Autodesk Inventor part; units mm, degrees
ref_plane "YZ Plane" through (0, 0, 0) normal (1, 0, 0) x (0, 1, 0)
ref_plane "XZ Plane" through (0, 0, 0) normal (0, 1, 0) x (-1, 0, 0)
ref_plane "XY Plane" through (0, 0, 0) normal (0, 0, 1) x (1, 0, 0)
sketch "Sketch1" plane through (0, 0, 0) normal (0, 0, 1) x (1, 0, 0)
  circle A0 centre (0, 0) radius 51.6188
  dimension "d0" = 103.2376
extrude "Extrusion1" add sketch "Sketch1" along normal mid plane 10
sketch "Sketch2" plane through (0, 0, 5) normal (0, 0, 1) x (1, 0, 0)
  circle A0 centre (0, 0) radius 51.6188
  arc A1 (-32.3092, 40.2568) -> (32.3092, 40.2568) centre (0, 73) ccw
  line L0 (0, 0) -> (36.5, 36.5) construction
  line L1 (0, -76.5426) -> (0, 97.9238) construction
  arc A2 (11.5258, 16.7584) -> (16.7584, 11.5258) centre (14.1421, 14.1421) ccw
  line L2 (11.5258, 16.7584) -> (33.7898, 39.0224)
  line L3 (16.7584, 11.5258) -> (39.0224, 33.7898)
  dimension "d3" = 46
  dimension "d4" = 73
  dimension "d5" = 20
  dimension "d6" = 45
  dimension "d7" = 3.7
extrude "Extrusion2" cut sketch "Sketch2" against normal through all contours L3 A2 L2 A0 | A0 A1
pattern_circular "Circular Pattern1" count 4 over 360 about axis through (0, 0, 0) along (0, 0, 1) of "Extrusion2"
chamfer "Chamfer1" distance 0.5 angle 45 8 edges at (0, 27, -5) (0, 27, 5) (27, 0, 5) (27, 0, -5) (-27, 0, 5) (0, -27, 5) (-27, 0, -5) (0, -27, -5)
sketch "Sketch3" plane through (0, 0, 5) normal (0, 0, 1) x (1, 0, 0)
  arc A0 (32.7, -39.9401) -> (-32.7, -39.9401) centre (0, -73) ccw
  line L0 (33.7898, -39.0224) -> (11.5258, -16.7584)
  arc A1 (16.7584, -11.5258) -> (11.5258, -16.7584) centre (14.1421, -14.1421) ccw
  line L1 (16.7584, -11.5258) -> (39.0224, -33.7898)
  arc A2 (39.9401, 32.7) -> (39.9401, -32.7) centre (73, 0) ccw
  line L2 (39.0224, 33.7898) -> (16.7584, 11.5258)
  arc A3 (11.5258, 16.7584) -> (16.7584, 11.5258) centre (14.1421, 14.1421) ccw
  line L3 (11.5258, 16.7584) -> (33.7898, 39.0224)
  arc A4 (-32.7, 39.9401) -> (32.7, 39.9401) centre (0, 73) ccw
  line L4 (-33.7898, 39.0224) -> (-11.5258, 16.7584)
  arc A5 (-16.7584, 11.5258) -> (-11.5258, 16.7584) centre (-14.1421, 14.1421) ccw
  line L5 (-16.7584, 11.5258) -> (-39.0224, 33.7898)
  arc A6 (-39.9401, -32.7) -> (-39.9401, 32.7) centre (-73, 0) ccw
  line L6 (-39.0224, -33.7898) -> (-16.7584, -11.5258)
  arc A7 (-11.5258, -16.7584) -> (-16.7584, -11.5258) centre (-14.1421, -14.1421) ccw
  line L7 (-11.5258, -16.7584) -> (-33.7898, -39.0224)
  line L8 (14.843, 22.904) -> (10.1116, 18.1726)
  arc A8 (10.1116, 18.1726) -> (18.1726, 10.1116) centre (14.1421, 14.1421) ccw
  line L9 (18.1726, 10.1116) -> (22.904, 14.843)
  arc A9 (26.2462, 12.8969) -> (26.2462, -12.8969) centre (73, 0) ccw
  line L10 (22.904, -14.843) -> (18.1726, -10.1116)
  arc A10 (18.1726, -10.1116) -> (10.1116, -18.1726) centre (14.1421, -14.1421) ccw
  line L11 (10.1116, -18.1726) -> (14.843, -22.904)
  arc A11 (12.8969, -26.2462) -> (-12.8969, -26.2462) centre (0, -73) ccw
  line L12 (-14.843, -22.904) -> (-10.1116, -18.1726)
  arc A12 (-10.1116, -18.1726) -> (-18.1726, -10.1116) centre (-14.1421, -14.1421) ccw
  line L13 (-18.1726, -10.1116) -> (-22.904, -14.843)
  arc A13 (-26.2462, -12.8969) -> (-26.2462, 12.8969) centre (-73, 0) ccw
  line L14 (-22.904, 14.843) -> (-18.1726, 10.1116)
  arc A14 (-18.1726, 10.1116) -> (-10.1116, 18.1726) centre (-14.1421, 14.1421) ccw
  line L15 (-10.1116, 18.1726) -> (-14.843, 22.904)
  arc A15 (-12.8969, 26.2462) -> (12.8969, 26.2462) centre (0, 73) ccw
  arc A16 (-12.8969, 26.2462) -> (-14.843, 22.904) centre (-13.4287, 24.3182) ccw
  arc A17 (14.843, 22.904) -> (12.8969, 26.2462) centre (13.4287, 24.3182) ccw
  arc A18 (26.2462, 12.8969) -> (22.904, 14.843) centre (24.3182, 13.4287) ccw
  arc A19 (22.904, -14.843) -> (26.2462, -12.8969) centre (24.3182, -13.4287) ccw
  arc A20 (12.8969, -26.2462) -> (14.843, -22.904) centre (13.4287, -24.3182) ccw
  arc A21 (-14.843, -22.904) -> (-12.8969, -26.2462) centre (-13.4287, -24.3182) ccw
  arc A22 (-26.2462, -12.8969) -> (-22.904, -14.843) centre (-24.3182, -13.4287) ccw
  arc A23 (-22.904, 14.843) -> (-26.2462, 12.8969) centre (-24.3182, 13.4287) ccw
  point P0 (21.4306, 29.4916)
  point P1 (29.4916, 21.4306)
  point P2 (29.4916, -21.4306)
  point P3 (21.4306, -29.4916)
  point P4 (-21.4306, -29.4916)
  point P5 (-29.4916, -21.4306)
  point P6 (-29.4916, 21.4306)
  point P7 (-21.4306, 29.4916)
  dimension "d16" = 2
  dimension "d17" = 2
extrude "Extrusion3" cut sketch "Sketch3" against normal blind 0.5
mirror "Mirror1" about plane through (0, 0, 0) normal (0, 0, 1) of "Extrusion3"
sketch "Sketch4" plane through (0, 0, 4.5) normal (0, 0, 1) x (1, 0, 0)
  circle A0 centre (0, 0) radius 9
  dimension "d20" = 18
extrude "Extrusion4" add sketch "Sketch4" along normal blind 10.5
sketch "Sketch5" plane through (0, 0, 15) normal (0, 0, 1) x (1, 0, 0)
  circle A0 centre (0, 0) radius 9
hole "Hole1" at (0, 0, 15) direction (0, 0, -1) diameter 9 end through all
fillet "Fillet1" radius 2 1 edges at (-9, 0, 4.5)
chamfer "Chamfer2" distance 1 angle 45 1 edges at (-9, 0, 15)
properties part number "Malta Cross" material "Steel"
Design review of the part built by this model. Coordinates are the model's own, in mm. A direction names the side the tool comes from. Coordinates: 2 decimals unless noted, no trailing zeros. Loops run counter-clockwise (first coordinate to the right, second up) from the corner with the lowest first, then second, coordinate; pieces in that order, holes last. Notation, with made-up numbers: M 26,34 L 31,34 A30 ccw 31,62 Z; hole C 37.5,63 d11. An arc over 180 degrees is marked long. Use one line per item in the form item = value.
(1) For faces 4 (the face through (-0.2, 24.5, 4.8)), 5 (the face through (15.175, -25.293, -4.754)), 6 (the face through (-27.73, -22.5, 0.07)), list the 3-axis set-ups (+Z, -Z, +X, -X, +Y, -Y) from which the entire face can be reached by the end or side of a thin tool; tool diameter is ignored.
Return value:
face_4 = +Z
face_5 = -Z
face_6 = +Z, -Z
(2) For line 1 along Y through (x, z) = (18.5, 1); line 2 along Y through (x, z) = (12.5, 1.5); line 3 along Z through (x, y) = (14, -7), list the stretches that pass through material, from the lowest coordinate up. Write a range as from..to.
Return value:
line_1 = -30.88..-23.73, -13.27..13.27, 23.73..30.88
line_2 = -28.73..-17.73, -10.83..10.83, 17.73..28.73
line_3 = -4.5..4.5
(3) Consider section A-A (y = 0). Write out the cut boundary in (x, z), and give its area (3 significant figures).
Return value:
outline = M -27,-4.5 L -26.5,-5 L -24.5,-5 L -24.5,-4.5 L -4.5,-4.5 L -4.5,15 L -8,15 L -9,14 L -9,6.5 A2 cw -11,4.5 L -24.5,4.5 L -24.5,5 L -26.5,5 L -27,4.5 Z; M 4.5,-4.5 L 24.5,-4.5 L 24.5,-5 L 26.5,-5 L 27,-4.5 L 27,4.5 L 26.5,5 L 24.5,5 L 24.5,4.5 L 11,4.5 A2 cw 9,6.5 L 9,14 L 8,15 L 4.5,15 Z
area = 505 mm2
(4) Draft analysis for pull direction X (two halves, no side actions). For faces 1 (the face through (20.505, -12.444, -4.754)), 2 (the face through (10.201, -10.024, 4.754)), 3 (the face through (-27.003, -0.501, 0.063)), state which applies: pulls with the +X half, pulls with the -X half, needs draft (parallel to the pull), parting line crosses it, or undercut.
Return value:
face_1 = undercut
face_2 = undercut
face_3 = pulls with the -X half
(5) Consider section C-C (z = -2.25). Write out the cut boundary in (x, y), and give its area (3 significant figures).
Return value:
outline = M -40.26,-32.31 A51.62 ccw -39.02,-33.79 L -16.76,-11.53 A3.7 cw -11.53,-16.76 L -33.79,-39.02 A51.62 ccw -32.31,-40.26 A46 cw 32.31,-40.26 A51.62 ccw 33.79,-39.02 L 11.53,-16.76 A3.7 cw 16.76,-11.53 L 39.02,-33.79 A51.62 ccw 40.26,-32.31 A46 cw 40.26,32.31 A51.62 ccw 39.02,33.79 L 16.76,11.53 A3.7 cw 11.53,16.76 L 33.79,39.02 A51.62 ccw 32.31,40.26 A46 cw -32.31,40.26 A51.62 ccw -33.79,39.02 L -11.53,16.76 A3.7 cw -16.76,11.53 L -39.02,33.79 A51.62 ccw -40.26,32.31 A46 cw Z; hole C 0,0 d9
area = 2,920 mm2
(6) Clearance check with flat-ended pins moving along their axes: P1, Ø12, axis at x = -6.5, y = -31.5, coming from the +Z side; P2, Ø10, axis at y = -1.5, z = 8, coming from the -X side; P3, Ø12, axis at x = 4, y = -7, coming from the -Z side. State where each tip first meets the part, or that it passes through.
Return value:
P1 = 5
P2 = -27.28
P3 = -4.5
